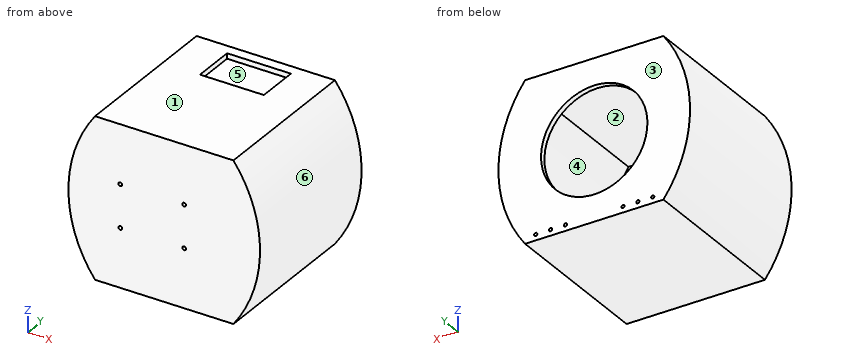
```python
from build123d import *

# Parameters (mm, degrees)
BOSS_EXTRUDE1_DEPTH      = 300
CUT_EXTRUDE8_DEPTH       = 280
COMPARTMENT_INPUT_R      = 100
CUT_EXTRUDE1_DEPTH       = 240
LCD_W                    = 120
LCD_H                    = 80
CUT_EXTRUDE2_DEPTH       = 10
HINGE_HOLES_R            = 3
CUT_EXTRUDE3_DEPTH       = 20
POLES_FOR_MIDDLE_LAYER_R = 17.5
BOSS_EXTRUDE2_DEPTH      = 110
HOLES_FOR_POLES_R        = 12.5
CUT_EXTRUDE6_DEPTH       = 50
CUT_EXTRUDE9_REACH       = 382.657
POWER_SUPPLY_HOLES_R     = 3.5


with BuildPart() as part:
    # Case 2 → Boss-Extrude1 (new body)
    with BuildSketch(Plane(origin=(0, 0, 0), x_dir=(1, 0, 0), z_dir=(0, 1, 0))):
        with BuildLine():
            Line((-130, 150), (130, 150))
            ThreePointArc((130, 150), (180, 0), (130, -150))
            Line((130, -150), (-130, -150))
            ThreePointArc((-130, -150), (-180, 0), (-130, 150))
        make_face()
    extrude(amount=BOSS_EXTRUDE1_DEPTH)

    # Hollow compartment → Cut-Extrude8 (cut)
    with BuildSketch(Plane(origin=(0, 290, 0), x_dir=(1, 0, 0), z_dir=(0, 1, 0))):
        with BuildLine():
            Line((-120, 130), (120, 130))
            ThreePointArc((120, 130), (158.257589982, 0), (120, -130))
            Line((120, -130), (-120, -130))
            ThreePointArc((-120, -130), (-158.257589982, 0), (-120, 130))
        make_face()
    extrude(amount=-CUT_EXTRUDE8_DEPTH, mode=Mode.SUBTRACT)

    # Compartment Input → Cut-Extrude1 (cut)
    with BuildSketch(Plane(origin=(0, 300, 0), x_dir=(1, 0, 0), z_dir=(0, 1, 0))):
        with Locations(Location((0, 0, 0), (0, 0, 270))):
            Circle(COMPARTMENT_INPUT_R)
    extrude(amount=-CUT_EXTRUDE1_DEPTH, mode=Mode.SUBTRACT)

    # LCD → Cut-Extrude2 (cut)
    with BuildSketch(Plane.XY.offset(150)):
        with Locations((0, 240)):
            Rectangle(LCD_W, LCD_H)
    extrude(amount=-CUT_EXTRUDE2_DEPTH, mode=Mode.SUBTRACT)

    # Hinge holes → Cut-Extrude3 (cut)
    with BuildSketch(Plane(origin=(0, 300, 0), x_dir=(1, 0, 0), z_dir=(0, 1, 0))):
        with Locations(Location((-110, 139, 0), (0, 0, 270))):
            Circle(HINGE_HOLES_R)
        with Locations(Location((-82, 139, 0), (0, 0, 270))):
            Circle(HINGE_HOLES_R)
        with Locations(Location((-54, 139, 0), (0, 0, 270))):
            Circle(HINGE_HOLES_R)
        with Locations(Location((54, 139, 0), (0, 0, 270))):
            Circle(HINGE_HOLES_R)
        with Locations(Location((82, 139, 0), (0, 0, 270))):
            Circle(HINGE_HOLES_R)
        with Locations(Location((110, 139, 0), (0, 0, 270))):
            Circle(HINGE_HOLES_R)
    extrude(amount=-CUT_EXTRUDE3_DEPTH, mode=Mode.SUBTRACT)

    # Poles for middle layer → Boss-Extrude2 (add)
    with BuildSketch(Plane(origin=(0, 10, 0), x_dir=(1, 0, 0), z_dir=(0, 1, 0))):
        with Locations(Location((0, 90, 0), (0, 0, 270))):
            Circle(POLES_FOR_MIDDLE_LAYER_R)
        with Locations(Location((0, -90, 0), (0, 0, 270))):
            Circle(POLES_FOR_MIDDLE_LAYER_R)
    extrude(amount=BOSS_EXTRUDE2_DEPTH)

    # Holes for poles → Cut-Extrude6 (cut)
    with BuildSketch(Plane(origin=(0, 120, 0), x_dir=(1, 0, 0), z_dir=(0, 1, 0))):
        with Locations(Location((0, -90, 0), (0, 0, 270))):
            Circle(HOLES_FOR_POLES_R)
        with Locations(Location((0, 90, 0), (0, 0, 270))):
            Circle(HOLES_FOR_POLES_R)
    extrude(amount=-CUT_EXTRUDE6_DEPTH, mode=Mode.SUBTRACT)

    # Power supply holes → Cut-Extrude9 (cut, up to next)
    with BuildSketch(Plane(origin=(0, 0, 0), x_dir=(1, 0, 0), z_dir=(0, 1, 0)), mode=Mode.PRIVATE) as cut_extrude9_sk1:
        with Locations(Location((-82.5, 40, 0), (0, 0, 90))):
            Circle(POWER_SUPPLY_HOLES_R)
    cut_extrude9_tool1 = extrude(cut_extrude9_sk1.sketch, amount=CUT_EXTRUDE9_REACH, mode=Mode.PRIVATE) & part.part
    # Power supply holes → Cut-Extrude9 (cut, up to next)
    with BuildSketch(Plane(origin=(0, 0, 0), x_dir=(1, 0, 0), z_dir=(0, 1, 0)), mode=Mode.PRIVATE) as cut_extrude9_sk2:
        with Locations(Location((37.5, 40, 0), (0, 0, 90))):
            Circle(POWER_SUPPLY_HOLES_R)
    cut_extrude9_tool2 = extrude(cut_extrude9_sk2.sketch, amount=CUT_EXTRUDE9_REACH, mode=Mode.PRIVATE) & part.part
    # Power supply holes → Cut-Extrude9 (cut, up to next)
    with BuildSketch(Plane(origin=(0, 0, 0), x_dir=(1, 0, 0), z_dir=(0, 1, 0)), mode=Mode.PRIVATE) as cut_extrude9_sk3:
        with Locations(Location((37.5, -40, 0), (0, 0, 90))):
            Circle(POWER_SUPPLY_HOLES_R)
    cut_extrude9_tool3 = extrude(cut_extrude9_sk3.sketch, amount=CUT_EXTRUDE9_REACH, mode=Mode.PRIVATE) & part.part
    # Power supply holes → Cut-Extrude9 (cut, up to next)
    with BuildSketch(Plane(origin=(0, 0, 0), x_dir=(1, 0, 0), z_dir=(0, 1, 0)), mode=Mode.PRIVATE) as cut_extrude9_sk4:
        with Locations(Location((-82.5, -40, 0), (0, 0, 90))):
            Circle(POWER_SUPPLY_HOLES_R)
    cut_extrude9_tool4 = extrude(cut_extrude9_sk4.sketch, amount=CUT_EXTRUDE9_REACH, mode=Mode.PRIVATE) & part.part
    add(cut_extrude9_tool1.solids().sort_by_distance((-82.5, 0, -40))[0], mode=Mode.SUBTRACT)
    add(cut_extrude9_tool2.solids().sort_by_distance((37.5, 0, -40))[0], mode=Mode.SUBTRACT)
    add(cut_extrude9_tool3.solids().sort_by_distance((37.5, 0, 40))[0], mode=Mode.SUBTRACT)
    add(cut_extrude9_tool4.solids().sort_by_distance((-82.5, 0, 40))[0], mode=Mode.SUBTRACT)


solid = part.part
```
Here's how the part is built. I have some questions about the finished solid (model axes, mm). Face numbers are marked on the shaded views. A direction names the side the tool comes from. Coordinates: 2 decimals unless noted, no trailing zeros. Loops run counter-clockwise (first coordinate to the right, second up) from the corner with the lowest first, then second, coordinate; pieces in that order, holes last. Notation, with made-up numbers: (67, -12) -> (122, -12) arc R21 cw to (122, 12) -> close; hole circle Ø7 at (48, 17.5). An arc over 180 degrees is marked (long way). Return JSON: item names as keys, results as strings.
1) I need wall thicknesses on line 1 (Z direction, x = -82.5, y = 4.75); line 2 (X direction, y = 73, z = 97); line 3 (Z direction, x = -20.5, y = 273.5). Which ranges of each line are inside material? Lowest first, please. Write a range as from..to.
Results below:
{"line 1": "-150..-43.5, -36.5..36.5, 43.5..150", "line 2": "-160.41..-137.78, -16.04..-10.36, 10.36..16.04, 137.78..160.41", "line 3": "-150..-130, 130..140"}
2) If we section it at A-A, the plane y = 92: Write out the boundary of the cut face in (x, z), then the cut area to 3 significant figures.
Results below:
{"outline": "(-130, -150) -> (130, -150) arc R250 ccw to (130, 150) -> (-130, 150) arc R250 ccw to start; circle Ø35 at (0, -90); circle Ø35 at (0, 90); hole (-120, -130) -> (120, -130) arc R240 ccw to (120, 130) -> (-120, 130) arc R240 ccw to start; hole circle Ø25 at (0, -90); hole circle Ø25 at (0, 90)", "area": "23,500 mm²"}
3) If we section it at D-D, the plane z = 0: Write out the boundary of the cut face in (x, y).
Results below:
{"outline": "(-180, 0) -> (180, 0) -> (180, 300) -> (100, 300) -> (100, 290) -> (158.26, 290) -> (158.26, 10) -> (-158.26, 10) -> (-158.26, 290) -> (-100, 290) -> (-100, 300) -> (-180, 300) -> close"}
4) Thinking about a two-plate mould opening in X: for the marked faces 3, 4, 5 and 6, which applies, +X half, -X half, draft (parallel to the pull), parting line (faces both ways), or undercut?
Results below:
{"face 3": "draft", "face 4": "undercut", "face 5": "undercut", "face 6": "+X half"}
5) For the marked faces 1 and 2, which set-ups out of +Z, -Z, +X, -X, +Y, -Y let a thin tool reach every point of the face, with its end or its side?
Results below:
{"face 1": "+Z, +X, -X, +Y, -Y", "face 2": "none"}
6) If we section it at B-B, the plane y = 177.5: Write out the boundary of the cut face in (x, z), then the cut area to 3 significant figures.
Results below:
{"outline": "(-130, -150) -> (130, -150) arc R250 ccw to (130, 150) -> (-130, 150) arc R250 ccw to start; hole (-120, -130) -> (120, -130) arc R240 ccw to (120, 130) -> (-120, 130) arc R240 ccw to start", "area": "22,500 mm²"}
7) If we section it at C-C, the plane z = 123: Write out the boundary of the cut face in (x, y), then the cut area to 3 significant figures.
Results below:
{"outline": "(-147.65, 0) -> (147.65, 0) -> (147.65, 300) -> (-147.65, 300) -> close; hole (-124.34, 10) -> (124.34, 10) -> (124.34, 290) -> (-124.34, 290) -> close", "area": "19,000 mm²"}
8) Will these pins go through, and if not, where does the flat tip stop? pin 1 (10.5 mm diameter, centred on x = 0.5, z = 84.5, fed in from +Y); pin 2 (12 mm diameter, centred on y = 105, z = 112, fed in from -X); pin 3 (8 mm diameter, centred on y = 155, z = 115, fed in from -X).
Results below:
{"pin 1": "y = 70", "pin 2": "x = -156.42", "pin 3": "x = -154.01"}
